Geometry check sheet. Reference: the model listing, model coordinates, mm. A direction names the side the tool comes from. Coordinates: 2 decimals unless noted, no trailing zeros. Write each loop counter-clockwise with the first axis right and the second up, starting at its lowest first coordinate (ties: lowest second). Pieces come first, ordered by that corner, then holes. Notation, with made-up numbers: (22, 18) - (40, 18) arc R20 ccw to (40, 46) - close; hole circle Ø4 at (6.5, 1.25). An arc over 180 degrees is marked (long way). Answer as a JSON object with one key per item and string values. Group by question number.
from build123d import *

# Parameters (mm, degrees)
SKETCH1_W           = 40
SKETCH1_H           = 40
BOSS_EXTRUDE1_DEPTH = 2
SKETCH2_R           = 1.5
CUT_EXTRUDE1_DEPTH  = 29.565713714
SKETCH3_W           = 4
SKETCH3_H           = 10
SKETCH3_W_2         = 10
SKETCH3_H_2         = 4
CUT_EXTRUDE2_DEPTH  = 29.565713714
SKETCH4_W           = 10
SKETCH4_H           = 4
BOSS_EXTRUDE2_DEPTH = 4
BOSS_EXTRUDE3_DEPTH = 4
SKETCH6_W           = 40
SKETCH6_H           = 26
CUT_EXTRUDE3_DEPTH  = 113.658776844
SKETCH7_W           = 4
SKETCH7_H           = 9
BOSS_EXTRUDE4_DEPTH = 4


with BuildPart() as part:
    # Sketch1 → Boss-Extrude1 (new, symmetric)
    with BuildSketch(Plane.XY):
        Rectangle(SKETCH1_W, SKETCH1_H)
    extrude(amount=BOSS_EXTRUDE1_DEPTH, both=True)

    # Sketch2 → Cut-Extrude1 (cut, through all)
    with BuildSketch(Plane.XY.offset(2)):
        with Locations((12, 14.35)):
            Circle(SKETCH2_R)
        with Locations((12, -3.15)):
            Circle(SKETCH2_R)
    extrude(amount=-CUT_EXTRUDE1_DEPTH, mode=Mode.SUBTRACT)

    # Sketch3 → Cut-Extrude2 (cut, through all)
    with BuildSketch(Plane.XY.offset(2)):
        with Locations((18, 10)):
            Rectangle(SKETCH3_W, SKETCH3_H)
        with Locations((-18, 10)):
            Rectangle(SKETCH3_W, SKETCH3_H)
        with Locations((-18, -10)):
            Rectangle(SKETCH3_W, SKETCH3_H)
        with Locations((18, -10)):
            Rectangle(SKETCH3_W, SKETCH3_H)
        with Locations((0, -8)):
            Rectangle(SKETCH3_W_2, SKETCH3_H_2)
    extrude(amount=-CUT_EXTRUDE2_DEPTH, mode=Mode.SUBTRACT)

    # Sketch4 → Boss-Extrude2 (add)
    with BuildSketch(Plane.XY.offset(2)):
        with Locations((-15, -22)):
            Rectangle(SKETCH4_W, SKETCH4_H)
        with Locations((15, -22)):
            Rectangle(SKETCH4_W, SKETCH4_H)
    extrude(amount=-BOSS_EXTRUDE2_DEPTH)

    # Sketch5 → Boss-Extrude3 (add)
    with BuildSketch(Plane.XY.offset(2)):
        Polygon((20, -20), (38, -20), (38, -24), (56, -24), (56, -20), (74, -20), (74, -24), (92, -24), (92, -20), (110, -20), (110, -10), (92, -10), (92, -6), (74, -6), (74, -10), (56, -10), (56, -6), (38, -6), (38, -10), (20, -10), align=None)
    extrude(amount=-BOSS_EXTRUDE3_DEPTH)

    # Sketch6 → Cut-Extrude3 (cut, through all)
    with BuildSketch(Plane.XY.offset(2)):
        with Locations((0, 7)):
            Rectangle(SKETCH6_W, SKETCH6_H)
    extrude(amount=-CUT_EXTRUDE3_DEPTH, mode=Mode.SUBTRACT)

    # Sketch7 → Boss-Extrude4 (add)
    with BuildSketch(Plane.XY.offset(2)):
        with Locations((18, -10.5)):
            Rectangle(SKETCH7_W, SKETCH7_H)
        with Locations((-18, -10.5)):
            Rectangle(SKETCH7_W, SKETCH7_H)
    extrude(amount=-BOSS_EXTRUDE4_DEPTH)


solid = part.part
(1) Material ranges on L1, parallel to X at y = -7.5, z = -0.8; L2, parallel to X at y = -21, z = -1.6; L3, parallel to Y at x = -8.5, z = 1.75, recorded low to high. Write a range as [from, to].
(2) Set-up check for faces 1 (the face through (0, -20, 0)), 2 (the face through (101, -20, 0)), 3 (the face through (38, -8, 0)): record each of +Z, -Z, +X, -X, +Y, -Y from which the full face is reachable in a straight line by a thin tool's end or side.
(3) Section check A-A (y = -7.75). Record the cut outline in (x, z).
(4) Gauge pin test, flat ends, axial feed: pin 1 (2 mm diameter, centred on y = -7, z = 0, fed in from +X); pin 2 (2 mm diameter, centred on x = -1.5, z = -0.5, fed in from +Y); pin 3 (1.5 mm diameter, centred on x = 94, y = -8.5, fed in from -Z). Record the tip position at first contact, or that the pin passes through.
(5) Section check C-C (x = 64). Record the cut outline in (y, z), and give its area (3 significant figures).
(6) Draft check along X on faces 4 (the face through (83, -24, 0)), 5 (the face through (92, -22, 0)), 6 (the face through (38, -22, 0)). Enter one of: +X half, -X half, draft (parallel to the pull), parting line (faces both ways), or undercut.
Conclusion:
{
 "1": {"L1": "x = [-20, -5], [5, 20], [38, 56], [74, 92]", "L2": "x = [-20, -10], [10, 20], [38, 56], [74, 92]", "L3": "y = [-20, -6]"},
 "2": {"face 1": "+Z, -Z, -Y", "face 2": "+Z, -Z, +X, -Y", "face 3": "+Z, -Z, +Y"},
 "3": {"outline": "(-20, -2) - (-5, -2) - (-5, 2) - (-20, 2) - close; (5, -2) - (20, -2) - (20, 2) - (5, 2) - close; (38, -2) - (56, -2) - (56, 2) - (38, 2) - close; (74, -2) - (92, -2) - (92, 2) - (74, 2) - close"},
 "4": {"pin 1": "stops at x = 92", "pin 2": "stops at y = -10", "pin 3": "passes through"},
 "5": {"outline": "(-20, -2) - (-10, -2) - (-10, 2) - (-20, 2) - close", "area": "40.0 mm^2"},
 "6": {"face 4": "draft", "face 5": "+X half", "face 6": "undercut"}
}
